from build123d import *

# Parameters (mm, degrees)
BOSS_EXTRUDE1_DEPTH = 3.175
SKETCH2_R           = 2.4638
SKETCH2_R_2         = 2.159
CUT_EXTRUDE1_DEPTH  = 4.175
SKETCH3_R           = 2.159
CUT_EXTRUDE2_DEPTH  = 4.175


with BuildPart() as part:
    # Sketch1 → Boss-Extrude1 (new body)
    with BuildSketch(Plane(origin=(0, 0, 0), x_dir=(1, 0, 0), z_dir=(0, 1, 0))):
        Polygon((-111.686526805, 95.25), (-127, 83.918625912), (-127, -83.918625912), (-111.686526805, -95.25), (111.686526805, -95.25), (127, -83.918625912), (127, 83.918625912), (111.686526805, 95.25), align=None)
        with BuildLine():
            Line((-107.95, -28.564963508), (-107.95, 28.564963508))
            ThreePointArc((-107.95, 28.564963508), (-104.304650999, 37.365614506), (-95.504, 41.010963508))
            Line((-95.504, 41.010963508), (-95.25, 41.010963508))
            Line((-95.25, 41.010963508), (-79.936526805, 52.342337595))
            Line((-79.936526805, 52.342337595), (-79.936526805, 63.754))
            ThreePointArc((-79.936526805, 63.754), (-76.291177804, 72.554650999), (-67.490526805, 76.2))
            Line((-67.490526805, 76.2), (67.490526805, 76.2))
            ThreePointArc((67.490526805, 76.2), (76.291177804, 72.554650999), (79.936526805, 63.754))
            Line((79.936526805, 63.754), (79.936526805, 52.342337595))
            Line((79.936526805, 52.342337595), (95.25, 41.010963508))
            Line((95.25, 41.010963508), (95.504, 41.010963508))
            ThreePointArc((95.504, 41.010963508), (104.304650999, 37.365614506), (107.95, 28.564963508))
            Line((107.95, 28.564963508), (107.95, -28.564963508))
            ThreePointArc((107.95, -28.564963508), (104.304650999, -37.365614506), (95.504, -41.010963508))
            Line((95.504, -41.010963508), (95.25, -41.010963508))
            Line((95.25, -41.010963508), (79.936526805, -52.342337595))
            Line((79.936526805, -52.342337595), (79.936526805, -63.754))
            ThreePointArc((79.936526805, -63.754), (76.291177804, -72.554650999), (67.490526805, -76.2))
            Line((67.490526805, -76.2), (-67.490526805, -76.2))
            ThreePointArc((-67.490526805, -76.2), (-76.291177804, -72.554650999), (-79.936526805, -63.754))
            Line((-79.936526805, -63.754), (-79.936526805, -52.342337595))
            Line((-79.936526805, -52.342337595), (-95.25, -41.010963508))
            Line((-95.25, -41.010963508), (-95.504, -41.010963508))
            ThreePointArc((-95.504, -41.010963508), (-104.304650999, -37.365614506), (-107.95, -28.564963508))
        make_face(mode=Mode.SUBTRACT)
    extrude(amount=BOSS_EXTRUDE1_DEPTH)

    # Sketch2 → Cut-Extrude1 (cut, through all)
    with BuildSketch(Plane(origin=(0, 3.175, 0), x_dir=(1, 0, 0), z_dir=(0, 1, 0))):
        with Locations((-95.147512794, 56.885632681)):
            Circle(SKETCH2_R)
        with Locations((-110.256011578, 77.303596941)):
            Circle(SKETCH2_R)
        with Locations((110.256011578, 77.303596941)):
            Circle(SKETCH2_R)
        with Locations((95.147512794, 56.885632681)):
            Circle(SKETCH2_R)
        with Locations((110.256011578, -77.303596941)):
            Circle(SKETCH2_R)
        with Locations((95.147512794, -56.885632681)):
            Circle(SKETCH2_R)
        with Locations((-110.256011578, -77.303596941)):
            Circle(SKETCH2_R)
        with Locations((-95.147512794, -56.885632681)):
            Circle(SKETCH2_R)
        with Locations((-88.154790208, 79.461855841)):
            Circle(SKETCH2_R_2)
        with Locations((-118.781736597, 56.799107666)):
            Circle(SKETCH2_R_2)
        with Locations((118.781736597, 56.799107666)):
            Circle(SKETCH2_R_2)
        with Locations((88.154790208, 79.461855841)):
            Circle(SKETCH2_R_2)
        with Locations((118.781736597, -56.799107666)):
            Circle(SKETCH2_R_2)
        with Locations((88.154790208, -79.461855841)):
            Circle(SKETCH2_R_2)
        with Locations((-88.154790208, -79.461855841)):
            Circle(SKETCH2_R_2)
        with Locations((-118.781736597, -56.799107666)):
            Circle(SKETCH2_R_2)
    extrude(amount=-CUT_EXTRUDE1_DEPTH, mode=Mode.SUBTRACT)

    # Sketch3 → Cut-Extrude2 (cut, through all)
    with BuildSketch(Plane(origin=(0, 3.175, 0), x_dir=(1, 0, 0), z_dir=(0, 1, 0))):
        with Locations((-76.2, 85.725)):
            Circle(SKETCH3_R)
        with Locations((-25.4, 85.725)):
            Circle(SKETCH3_R)
        with Locations((25.4, 85.725)):
            Circle(SKETCH3_R)
        with Locations((76.2, 85.725)):
            Circle(SKETCH3_R)
        with Locations((76.2, -85.725)):
            Circle(SKETCH3_R)
        with Locations((25.4, -85.725)):
            Circle(SKETCH3_R)
        with Locations((-25.4, -85.725)):
            Circle(SKETCH3_R)
        with Locations((-76.2, -85.725)):
            Circle(SKETCH3_R)
        with Locations((-117.475, -25.4)):
            Circle(SKETCH3_R)
        with Locations((-117.475, 25.4)):
            Circle(SKETCH3_R)
        with Locations((117.475, 25.4)):
            Circle(SKETCH3_R)
        with Locations((117.475, -25.4)):
            Circle(SKETCH3_R)
        with Locations((0, 85.725)):
            Circle(SKETCH3_R)
        with Locations((0, -85.725)):
            Circle(SKETCH3_R)
        with Locations((-117.475, 0)):
            Circle(SKETCH3_R)
        with Locations((117.475, 0)):
            Circle(SKETCH3_R)
    extrude(amount=-CUT_EXTRUDE2_DEPTH, mode=Mode.SUBTRACT)


solid = part.part
Geometry: final body of the model. Coordinates: model frame, mm. A direction names the side the tool comes from. Give positions to 0.01 mm unless a question says otherwise; leave off trailing zeros. Loops run counter-clockwise (first coordinate to the right, second up) from the corner with the lowest first, then second, coordinate; pieces in that order, holes last. Notation, with made-up numbers: M -36,51.5 L -3,51.5 A22 ccw -3,82.5 Z; hole C 27.25,43.25 d6. An arc over 180 degrees is marked long. Put each result on its own line as item: value. Start each with the question number.
1) Cut plane A-A (z = 16). Output: boundary loops of the cut face in (x, y) (3 decimals), then the cut area to 3 significant figures.
2) Contact query for a flat-ended pin moving along its axis: pin 1 (4 mm diameter, centred on x = 118.78, z = -56.8, fed in from -Y). Output: stop coordinate, or through.
3) Cut plane C-C (y = 1.7). Give the number of separate pieces and of enclosed holes in the cut face, then the cut area to 3 significant figures.
4) Ray query, line 1 along X through (y, z) = (0.8, 0); line 2 along Z through (x, y) = (-51, 2.5); line 3 along X through (y, z) = (2.2, 63.5). Return the intervals inside material, ascending.
5) Cut plane B-B (x = 12.5). Output: boundary loops of the cut face in (y, z) (3 decimals).
6) Access query for faces 1 (the cylindrical face through (-104.21, 1.57, 37.46)), 2 (the flat face through (-119.24, 1.57, -89.66)). Directions: +Z, -Z, +X, -X, +Y, -Y. A direction counts if a zero-diameter tool reaches every point of the face in a straight line with its end or side. Return the directions, or none.
Verdict:
1. outline: M -127,0 L -107.95,0 L -107.95,3.175 L -127,3.175 Z; M 107.95,0 L 127,0 L 127,3.175 L 107.95,3.175 Z
1. area: 121 mm2
2. pin 1: through
3. separate pieces: 1
3. enclosed holes: 33
3. area: 18,500 mm2
4. line 1: -127 to -119.63, -115.32 to -107.95, 107.95 to 115.32, 119.63 to 127
4. line 2: -95.25 to -76.2, 76.2 to 95.25
4. line 3: -127 to -79.94, 79.94 to 127
5. outline: M 0,-95.25 L 3.175,-95.25 L 3.175,-76.2 L 0,-76.2 Z; M 0,76.2 L 3.175,76.2 L 3.175,95.25 L 0,95.25 Z
6. face 1: +Y, -Y
6. face 2: -Z, -X, +Y, -Y
